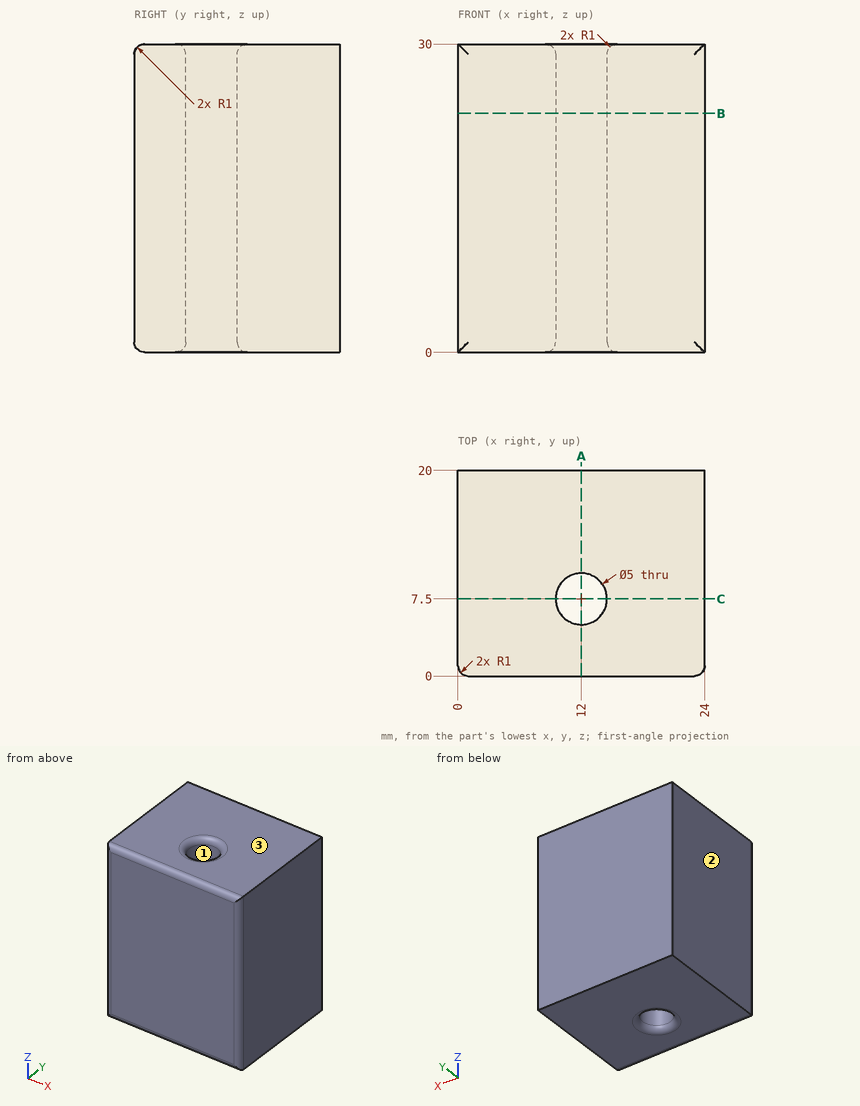
Design review of the part shown in the three views and the two pictorial views. Dimensions are in mm from the part's minimum x, y and z. Round coordinates to 2 decimals unless told otherwise and drop trailing zeros. Loops run counter-clockwise (first coordinate to the right, second up) from the corner with the lowest first, then second, coordinate; pieces in that order, holes last. Notation, with made-up numbers: (17, 8.25) - (68, 8.25) arc R16 ccw to (68, 25.25) - close; hole circle Ø10 at (45, -18.5). An arc over 180 degrees is marked (long way). One line per item, written item: value. Start each with the question number.
Item 1: The part is to be moulded in two halves that separate along X. For the marked faces 1, 2 and 3, say which applies: +X half, -X half, draft (parallel to the pull), parting line (faces both ways), or undercut.
Item 2: Clearance check with flat-ended pins moving along their axes: pin 1 Ø3 at (x, y) = (12.5, 9) entering from -Z; pin 2 Ø5 at (x, y) = (18, 11.5) entering from -Z; pin 3 Ø3 at (x, y) = (12, 7.5) entering from +Z. State where each tip first meets the part, or that it passes through.
Item 3: Take a section at C-C (y = 7.5). Give the boundary of the cut face in (x, z).
Item 4: For L1, parallel to X at y = 7.5, z = 9.75; L2, parallel to Y at x = 12, z = 22.25; L3, parallel to Y at x = 10, z = 14, list the stretches that pass through material, from the lowest coordinate up.
Item 5: Take a section at A-A (x = 12). Give the boundary of the cut face in (y, z).
Item 6: Take a section at B-B (z = 23.25). Give the boundary of the cut face in (x, y), plus the area to 3 significant figures.
Answer below:
1. face 1: undercut
1. face 2: -X half
1. face 3: draft
2. pin 1: stops at z = 0.09
2. pin 2: stops at z = 0
2. pin 3: passes through
3. outline: (0, 0) - (8.5, 0) arc R1 ccw to (9.5, 1) - (9.5, 29) arc R1 ccw to (8.5, 30) - (0, 30) - close; (14.5, 1) arc R1 ccw to (15.5, 0) - (24, 0) - (24, 30) - (15.5, 30) arc R1 ccw to (14.5, 29) - close
4. L1: x = 0 to 9.5, 14.5 to 24
4. L2: y = 0 to 5, 10 to 20
4. L3: y = 0 to 6, 9 to 20
5. outline: (0, 1) arc R1 ccw to (1, 0) - (4, 0) arc R1 ccw to (5, 1) - (5, 29) arc R1 ccw to (4, 30) - (1, 30) arc R1 ccw to (0, 29) - close; (10, 1) arc R1 ccw to (11, 0) - (20, 0) - (20, 30) - (11, 30) arc R1 ccw to (10, 29) - close
6. outline: (0, 1) arc R1 ccw to (1, 0) - (23, 0) arc R1 ccw to (24, 1) - (24, 20) - (0, 20) - close; hole circle Ø5 at (12, 7.5)
6. area: 460 mm2
